Geometry check sheet. Reference: drawing and pictorial views, mm from the part's lowest x, y, z. A direction names the side the tool comes from. Give positions to 0.01 mm unless a question says otherwise; leave off trailing zeros. Write each loop counter-clockwise with the first axis right and the second up, starting at its lowest first coordinate (ties: lowest second). Pieces come first, ordered by that corner, then holes.
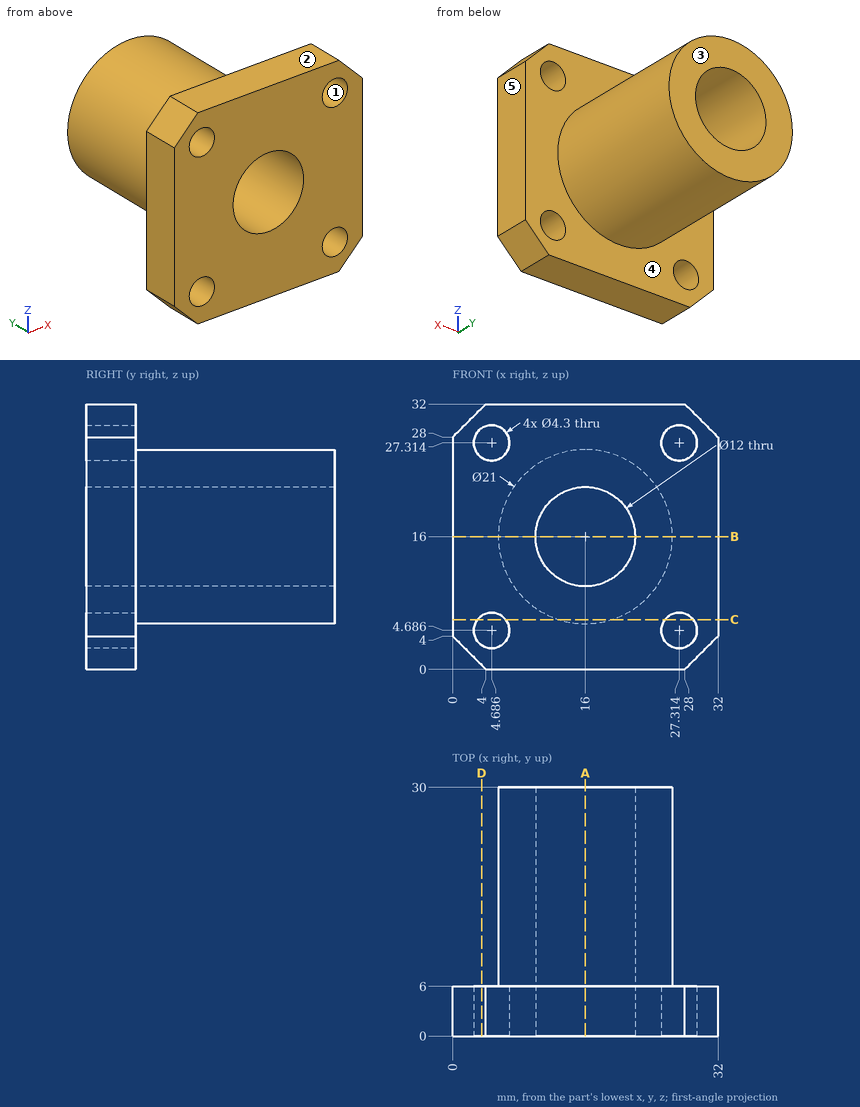
Item 1: Depth check by flat-ended pin: pin 1 (12 mm diameter, centred on x = 15, y = 16.5, fed in from +Z); pin 2 (2 mm diameter, centred on y = 12.5, z = 14, fed in from -X); pin 3 (4 mm diameter, centred on x = 16, y = 19.5, fed in from -Z). Enter the tip coordinate at first touch or a pass-through.
Answer key:
pin 1: stops at z = 26.5
pin 2: stops at x = 5.55
pin 3: stops at z = 5.5
Item 2: Sectioned sample at D-D on x = 3.5. Record the cut outline in (y, z).
Answer key:
outline: (0, 0.5) - (6, 0.5) - (6, 2.89) - (0, 2.89) - close; (0, 6.48) - (6, 6.48) - (6, 25.52) - (0, 25.52) - close; (0, 29.11) - (6, 29.11) - (6, 31.5) - (0, 31.5) - close
Item 3: Sectioned sample at A-A on x = 16. Record the cut outline in (y, z), then the cut area to 3 significant figures.
Answer key:
outline: (0, 0) - (6, 0) - (6, 5.5) - (30, 5.5) - (30, 10) - (0, 10) - close; (0, 22) - (30, 22) - (30, 26.5) - (6, 26.5) - (6, 32) - (0, 32) - close
area: 336 mm2
Item 4: Sectioned sample at C-C on z = 6. Record the cut outline in (x, y).
Answer key:
outline: (0, 0) - (2.98, 0) - (2.98, 6) - (0, 6) - close; (6.39, 0) - (25.61, 0) - (25.61, 6) - (19.2, 6) - (19.2, 30) - (12.8, 30) - (12.8, 6) - (6.39, 6) - close; (29.02, 0) - (32, 0) - (32, 6) - (29.02, 6) - close
Item 5: Scan lines: line 1 along Y through (x, z) = (27, 22); line 2 along X through (y, z) = (7, 12); line 3 along X through (y, z) = (26.5, 13) (1 decimal). Record each from-to range of solid material in increasing order.
Answer key:
line 1: y = 0 to 6
line 2: x = 6.29 to 11.53, 20.47 to 25.71
line 3: x = 5.9 to 10.8, 21.2 to 26.1
Item 6: Sectioned sample at B-B on z = 16. Record the cut outline in (x, y), then the cut area to 3 significant figures.
Answer key:
outline: (0, 0) - (10, 0) - (10, 30) - (5.5, 30) - (5.5, 6) - (0, 6) - close; (22, 0) - (32, 0) - (32, 6) - (26.5, 6) - (26.5, 30) - (22, 30) - close
area: 336 mm2
Item 7: Set-up check for the marked faces 4 and 5: record each of +Z, -Z, +X, -X, +Y, -Y from which the full face is reachable in a straight line by a thin tool's end or side.
Answer key:
face 4: +Y
face 5: +Z, -Z, +X, +Y, -Y
Item 8: Release check for a two-part mould opening along Z. For the marked faces 1, 2 and 3 record: released by +Z, released by -Z, zero draft, split by the parting line, or undercut.
Answer key:
face 1: undercut
face 2: released by +Z
face 3: zero draft
